Geometry check sheet. Reference: the model listing, model coordinates, mm. A direction names the side the tool comes from. Round coordinates to 2 decimals unless told otherwise and drop trailing zeros. Loops run counter-clockwise (first coordinate to the right, second up) from the corner with the lowest first, then second, coordinate; pieces in that order, holes last. Notation, with made-up numbers: (62.25, -21) - (108.25, -21) arc R23 cw to (108.25, -13) - close; hole circle Ø4 at (-15.75, 45.5). An arc over 180 degrees is marked (long way). Write item = value, one per line.
```python
from build123d import *

# Parameters (mm, degrees)
SKETCH1_W            = 68.987924
SKETCH1_H            = 80.264
BOSS_EXTRUDE3_DEPTH  = 2.54
SKETCH1_7_W          = 63.907924
SKETCH1_7_H          = 77.724
BOSS_EXTRUDE4_DEPTH  = 2.54
SKETCH1_9_W          = 46.99
SKETCH1_9_H          = 1.27
BOSS_EXTRUDE6_DEPTH  = 15.748
SKETCH2_W            = 6.35
SKETCH2_H            = 22.098
CUT_EXTRUDE1_DEPTH   = 2.54
SKETCH3_W            = 16.917924
SKETCH3_H            = 1.27
BOSS_EXTRUDE7_DEPTH  = 6.35
SKETCH4_W            = 21.336
SKETCH4_H            = 32.512
CUT_EXTRUDE2_DEPTH   = 5.08
SKETCH5_W            = 25.4
SKETCH5_H            = 31.75
CUT_EXTRUDE3_DEPTH   = 5.08
SKETCH5_3_W          = 26.924
SKETCH5_3_H          = 33.34449199
SKETCH5_3_W_2        = 25.4
SKETCH5_3_H_2        = 31.75
BOSS_EXTRUDE8_DEPTH  = 12.7
BOSS_EXTRUDE9_START  = 12.7
SKETCH5_4_W          = 25.4
SKETCH5_4_H          = 31.75
BOSS_EXTRUDE9_DEPTH  = 1.27
SKETCH7_W            = 22.86
SKETCH7_H            = 34.036
SKETCH7_W_2          = 21.336
SKETCH7_H_2          = 32.512
BOSS_EXTRUDE10_DEPTH = 5.334
SKETCH6_W            = 6.35
SKETCH6_H            = 33.02
CUT_EXTRUDE5_DEPTH   = 5.334
SKETCH9_W            = 43.18
SKETCH9_H            = 2.54
BOSS_EXTRUDE12_DEPTH = 12.827
SKETCH10_W           = 2.54
SKETCH10_H           = 8.128
BOSS_EXTRUDE13_DEPTH = 32.258
BOSS_EXTRUDE14_DEPTH = 8.128


with BuildPart() as part:
    # Sketch1 → Boss-Extrude3 (new body)
    with BuildSketch(Plane(origin=(0, 0, 0), x_dir=(0, 0, -1), z_dir=(1, 0, 0))):
        with Locations((0.050038, -1.397)):
            Rectangle(SKETCH1_W, SKETCH1_H)
    extrude(amount=BOSS_EXTRUDE3_DEPTH)

    # Sketch1<7> → Boss-Extrude4 (add)
    with BuildSketch(Plane(origin=(0, 0, 0), x_dir=(0, 0, -1), z_dir=(1, 0, 0))):
        with Locations((0.050038, -0.127)):
            Rectangle(SKETCH1_7_W, SKETCH1_7_H)
    extrude(amount=-BOSS_EXTRUDE4_DEPTH)

    # Sketch1<9> → Boss-Extrude6 (add)
    with BuildSketch(Plane(origin=(0, 0, 0), x_dir=(0, 0, -1), z_dir=(1, 0, 0))):
        with Locations((-8.408924, 38.1)):
            Rectangle(SKETCH1_9_W, SKETCH1_9_H)
    extrude(amount=-BOSS_EXTRUDE6_DEPTH)

    # Sketch2 → Cut-Extrude1 (cut)
    with BuildSketch(Plane(origin=(0, 38.735, 0), x_dir=(1, 0, 0), z_dir=(0, 1, 0))):
        with Locations((-8.763, -10.567924)):
            Rectangle(SKETCH2_W, SKETCH2_H)
    extrude(amount=-CUT_EXTRUDE1_DEPTH, mode=Mode.SUBTRACT)

    # Sketch3 → Boss-Extrude7 (add)
    with BuildSketch(Plane.ZY.offset(2.54)):
        with Locations((-23.545038, 38.1)):
            Rectangle(SKETCH3_W, SKETCH3_H)
    extrude(amount=BOSS_EXTRUDE7_DEPTH)

    # Sketch4 → Cut-Extrude2 (cut)
    with BuildSketch(Plane(origin=(2.54, 0, 0), x_dir=(0, 0, -1), z_dir=(1, 0, 0))):
        with Locations((-10.313924, 11.303)):
            Rectangle(SKETCH4_W, SKETCH4_H)
    extrude(amount=-CUT_EXTRUDE2_DEPTH, mode=Mode.SUBTRACT)

    # Sketch5 → Cut-Extrude3 (cut)
    with BuildSketch(Plane(origin=(2.54, 0, 0), x_dir=(0, 0, -1), z_dir=(1, 0, 0))):
        with Locations((13.816076, 17.526)):
            Rectangle(SKETCH5_W, SKETCH5_H)
    extrude(amount=-CUT_EXTRUDE3_DEPTH, mode=Mode.SUBTRACT)

    # Sketch5<3> → Boss-Extrude8 (add)
    with BuildSketch(Plane(origin=(2.54, 0, 0), x_dir=(0, 0, -1), z_dir=(1, 0, 0))):
        with Locations((13.816076, 17.526)):
            Rectangle(SKETCH5_3_W, SKETCH5_3_H)
        with Locations((13.816076, 17.526)):
            Rectangle(SKETCH5_3_W_2, SKETCH5_3_H_2, mode=Mode.SUBTRACT)
    extrude(amount=BOSS_EXTRUDE8_DEPTH)

    # Sketch5<4> → Boss-Extrude9 (add)
    with BuildSketch(Plane(origin=(2.54, 0, 0), x_dir=(0, 0, -1), z_dir=(1, 0, 0)).offset(BOSS_EXTRUDE9_START)):
        with Locations((13.816076, 17.526)):
            Rectangle(SKETCH5_4_W, SKETCH5_4_H)
    extrude(amount=-BOSS_EXTRUDE9_DEPTH)

    # Sketch7 → Boss-Extrude10 (add)
    with BuildSketch(Plane.ZY.offset(2.54)):
        with Locations((10.313924, 11.303)):
            Rectangle(SKETCH7_W, SKETCH7_H)
        with Locations((10.313924, 11.303)):
            Rectangle(SKETCH7_W_2, SKETCH7_H_2, mode=Mode.SUBTRACT)
    extrude(amount=BOSS_EXTRUDE10_DEPTH)

    # Sketch6 → Cut-Extrude5 (cut)
    with BuildSketch(Plane.ZY.offset(2.54)):
        with Locations((-19.531076, -17.399)):
            Rectangle(SKETCH6_W, SKETCH6_H)
    extrude(amount=-CUT_EXTRUDE5_DEPTH, mode=Mode.SUBTRACT)

    # Sketch9 → Boss-Extrude12 (add)
    with BuildSketch(Plane.ZY.offset(2.54)):
        with Locations((10.313924, -37.719)):
            Rectangle(SKETCH9_W, SKETCH9_H)
    extrude(amount=BOSS_EXTRUDE12_DEPTH)

    # Sketch10 → Boss-Extrude13 (add)
    with BuildSketch(Plane.ZY.offset(-13.97)):
        with Locations((-12.444476, 27.686)):
            Rectangle(SKETCH10_W, SKETCH10_H)
    extrude(amount=BOSS_EXTRUDE13_DEPTH)

    # Sketch11 → Boss-Extrude14 (add)
    with BuildSketch(Plane(origin=(0, 31.75, 0), x_dir=(1, 0, 0), z_dir=(0, 1, 0))):
        with BuildLine():
            Line((-18.288, 13.714476), (-18.288, 8.951976))
            Line((-18.288, 8.951976), (-21.272654916, 12.682794645))
            ThreePointArc((-21.272654916, 12.682794645), (-21.349130777, 13.354550844), (-20.776803222, 13.714476))
            Line((-20.776803222, 13.714476), (-18.288, 13.714476))
        make_face()
    extrude(amount=-BOSS_EXTRUDE14_DEPTH)


solid = part.part
```
(1) Section check A-A (x = -6.5). Enter the section's corners in (y, z) (3 decimals).
Answers follow:
outline = (-38.989, -11.276) - (-36.449, -11.276) - (-36.449, 31.904) - (-38.989, 31.904) - close; (-5.715, -1.116) - (28.321, -1.116) - (28.321, 21.744) - (-5.715, 21.744) - close; (23.622, -13.714) - (31.75, -13.714) - (31.75, -11.174) - (23.622, -11.174) - close; (37.465, -32.004) - (38.735, -32.004) - (38.735, -0.481) - (37.465, -0.481) - close; (37.465, 21.617) - (38.735, 21.617) - (38.735, 31.904) - (37.465, 31.904) - close; hole (-4.953, -0.354) - (27.559, -0.354) - (27.559, 20.982) - (-4.953, 20.982) - close
(2) Section check C-C (y = -31). Enter the section's corners in (x, z).
Answers follow:
outline = (-2.54, -32) - (0, -32) - (0, -34.54) - (2.54, -34.54) - (2.54, -22.71) - (-2.54, -22.71) - close; (-2.54, -16.36) - (2.54, -16.36) - (2.54, 34.44) - (0, 34.44) - (0, 31.9) - (-2.54, 31.9) - close
(3) Scan lines: L1, parallel to Z at x = 11, y = 29.5; L2, parallel to Z at x = -4, y = 7.5; L3, parallel to Y at x = -14, z = 1 (3 decimals). Record each from-to range of solid material in increasing order. Write a range as [from, to].
Answers follow:
L1 = [-27.28, -26.52], [-13.71, -11.17], [-1.12, -0.35]
L2 = [-1.12, -0.35], [20.98, 21.74]
L3 = [-38.989, -36.449], [37.465, 38.735]
(4) Section check B-B (x = 6). Enter the section's corners in (y, z), then the cut area to 3 significant figures.
Answers follow:
outline = (0.85, -27.28) - (34.2, -27.28) - (34.2, -0.35) - (0.85, -0.35) - close; (23.62, -13.71) - (31.75, -13.71) - (31.75, -11.17) - (23.62, -11.17) - close; hole (1.65, -26.52) - (33.4, -26.52) - (33.4, -1.12) - (1.65, -1.12) - close
area = 112 mm²
(5) Set-up check for faces 5 (the flat face through (9, 34.198, -14)), 6 (the flat face through (0, -0.889, -20)), 7 (the flat face through (-3, 23.622, -12)): record each of +Z, -Z, +X, -X, +Y, -Y from which the full face is reachable in a straight line by a thin tool's end or side.
Answers follow:
face_5 = +Z, -Z, +X, +Y
face_6 = +X, -X
face_7 = -X
(6) Mould release check, pull along Y, two halves, no side actions. Record for faces 1 (the flat face through (1, -41.529, 0)), 2 (the flat face through (15.24, 18, -14)), 3 (the flat face through (-5, 11, 21.744)), 4 (the flat face through (-2, 28, -11.174)): pulls with the +Y half, pulls with the -Y half, needs draft (parallel to the pull), parting line crosses it, or undercut.
Answers follow:
face_1 = pulls with the -Y half
face_2 = needs draft
face_3 = undercut
face_4 = undercut
(7) Section check D-D (z = 17.5). Enter the section's corners in (x, y) (3 decimals), then the cut area to 3 significant figures.
Answers follow:
outline = (-15.748, 37.465) - (-11.938, 37.465) - (-11.938, 38.735) - (-15.748, 38.735) - close; (-15.367, -38.989) - (0, -38.989) - (0, -41.529) - (2.54, -41.529) - (2.54, -4.953) - (-7.874, -4.953) - (-7.874, -5.715) - (-2.54, -5.715) - (-2.54, -36.449) - (-15.367, -36.449) - close; (-7.874, 27.559) - (2.54, 27.559) - (2.54, 38.735) - (-5.588, 38.735) - (-5.588, 37.465) - (-2.54, 37.465) - (-2.54, 28.321) - (-7.874, 28.321) - close
area = 286 mm²
(8) Gauge pin test, flat ends, axial feed: pin 1 (17 mm diameter, centred on x = -11, z = 0, fed in from -Y); pin 2 (5 mm diameter, centred on x = 8, y = 18.5, fed in from +Z); pin 3 (1.5 mm diameter, centred on x = 3.5, z = -24, fed in from +Y). Record the tip position at first contact, or that the pin passes through.
Answers follow:
pin_1 = -38.99
pin_2 = -0.35
pin_3 = 34.2
